Verification items for this drawing (mm, ordinates from the low corner). A direction names the side the tool comes from. Round coordinates to 2 decimals unless told otherwise and drop trailing zeros. Loops run counter-clockwise (first coordinate to the right, second up) from the corner with the lowest first, then second, coordinate; pieces in that order, holes last. Notation, with made-up numbers: (-28, 55.25) - (29, 55.25) arc R33 ccw to (29, 86.25) - close; hole circle Ø7 at (-11, -21.5). An arc over 180 degrees is marked (long way). Answer in a Markdown table with one row per item. Add a question column.
(1) Access from +Z, -Z, +X, -X, +Y, -Y to the whole of each face (thin tool, end or side, straight path). Record for the marked faces 1 and 2.
(2) Cross-section at D-D on y = 7.5. Enter the section's corners in (x, z), then the cut area to 3 significant figures.
(3) Gauge pin test, flat end, axial feed: pin 1 (1 mm diameter, centred on x = 2.5, y = 6.5, fed in from +Z). Record the tip position at first contact, or that the pin passes through.
(4) Cross-section at B-B on y = 9. Enter the section's corners in (x, z), then the cut area to 3 significant figures.
(5) Cross-section at A-A on x = 12. Enter the section's corners in (y, z), then the cut area to 4 significant figures.
(6) Cross-section at C-C on x = 16.25. Enter the section's corners in (y, z), then the cut area to 3 significant figures.
(7) Thickness scan on line 1 along Z through (x, y) = (11, 9.5); line 2 along Z through (x, y) = (11, 3.25); line 3 along X through (y, z) = (2.25, 24). Record the ranges inside material, lowest first.
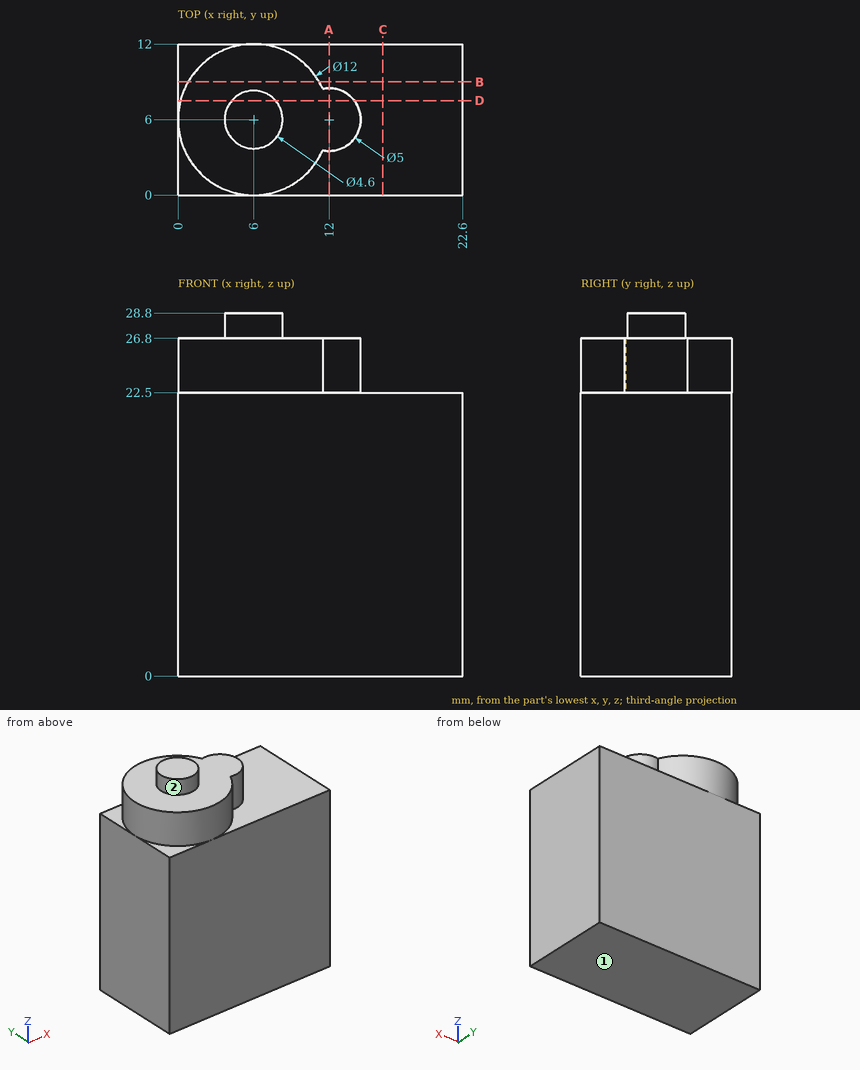
Answers:
| question | item | result |
|---|---|---|
| 1 | face 1 | -Z, +X, -X, +Y, -Y |
| 1 | face 2 | +Z |
| 2 | outline | (0, 0) - (22.6, 0) - (22.6, 22.5) - (14, 22.5) - (14, 26.8) - (7.74, 26.8) - (7.74, 28.8) - (4.26, 28.8) - (4.26, 26.8) - (0.19, 26.8) - (0.19, 22.5) - (0, 22.5) - close |
| 2 | area | 575 mm^2 |
| 3 | pin 1 | stops at z = 26.8 |
| 4 | outline | (0, 0) - (22.6, 0) - (22.6, 22.5) - (11.2, 22.5) - (11.2, 26.8) - (0.8, 26.8) - (0.8, 22.5) - (0, 22.5) - close |
| 4 | area | 553 mm^2 |
| 5 | outline | (0, 0) - (12, 0) - (12, 22.5) - (8.5, 22.5) - (8.5, 26.8) - (3.5, 26.8) - (3.5, 22.5) - (0, 22.5) - close |
| 5 | area | 291.5 mm^2 |
| 6 | outline | (0, 0) - (12, 0) - (12, 22.5) - (0, 22.5) - close |
| 6 | area | 270 mm^2 |
| 7 | line 1 | z = 0 to 22.5 |
| 7 | line 2 | z = 0 to 26.8 |
| 7 | line 3 | x = 1.32 to 10.68 |
